Part model, mm, in its own coordinate system. Face numbers are marked on the shaded views. Give positions to 0.01 mm unless a question says otherwise; leave off trailing zeros. Order: outer loops, then holes, each group sorted by start corner. A loop starts at its lowest first (then second) coordinate and runs counter-clockwise, first axis right, second up. Notation, with made-up numbers: M -4.5,-12.5 L 17.5,-12.5 A22 cw 17.5,12.5 Z; hole C -12.75,-33.5 d10. An arc over 180 degrees is marked long. One line per question, with ' | ' between items.
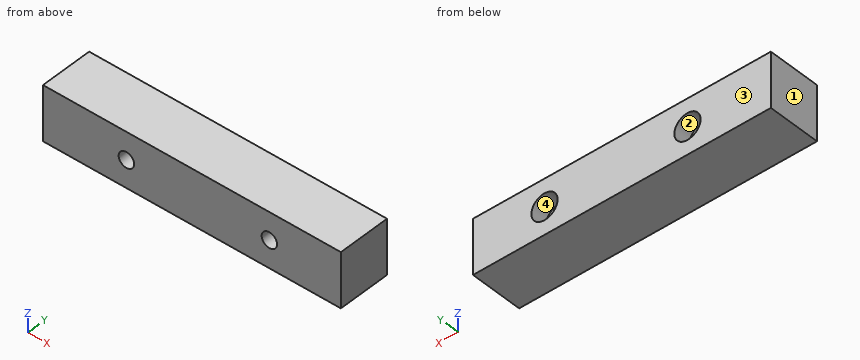
```python
from build123d import *

# Parameters (mm, degrees)
SKETCH_1_W                = 23
SKETCH_1_H                = 22
EXTRUDE_1_DEPTH           = 125
HOLE_WIZARD_1_D           = 6.5
HOLE_WIZARD_1_CBORE_D     = 11
HOLE_WIZARD_1_CBORE_DEPTH = 7
PATTERN_LINEAR_2_COUNT    = 2
PATTERN_LINEAR_2_PITCH    = 60


with BuildPart() as part:
    # 草图1 → 凸台-拉伸1 (new body)
    with BuildSketch(Plane(origin=(0, 0, 0), x_dir=(0, 0, -1), z_dir=(1, 0, 0))):
        Rectangle(SKETCH_1_W, SKETCH_1_H)
    extrude(amount=EXTRUDE_1_DEPTH)

    # 打孔尺寸(%根据)内六角圆柱头螺钉的类型1 (through all)
    with Locations(Plane(origin=(0, 11, 0), x_dir=(1, 0, 0), z_dir=(0, 1, 0))):
        with Locations((35, 0)):
            hole_wizard_1 = CounterBoreHole(HOLE_WIZARD_1_D / 2, HOLE_WIZARD_1_CBORE_D / 2, HOLE_WIZARD_1_CBORE_DEPTH)

    # 阵列(线性)2: 打孔尺寸(%根据)内六角圆柱头螺钉的类型1 ×2
    with Locations(*[(i * PATTERN_LINEAR_2_PITCH, 0, 0) for i in range(1, PATTERN_LINEAR_2_COUNT)]):
        add(hole_wizard_1, mode=Mode.SUBTRACT)


solid = part.part
```
1. Slice it at B-B on y = -5.5. Give the cut face in (x, z), then the cut area to 3 significant figures.
Worked out:
outline: M 0,-11.5 L 125,-11.5 L 125,11.5 L 0,11.5 Z; hole C 35,0 d6.5; hole C 95,0 d6.5 | area: 2,810 mm2
2. Probe L1, parallel to Z at x = 95, y = 9; L2, parallel to X at y = 5.25, z = -4.75; L3, parallel to X at y = -1, z = 0.75. List the from-to ranges inside material, lowest first. Write a range as from..to.
Worked out:
L1: z = -11.5..-5.5, 5.5..11.5 | L2: x = 0..32.23, 37.77..92.23, 97.77..125 | L3: x = 0..31.84, 38.16..91.84, 98.16..125
3. Drop a flat-ended pin along its axis: pin 1 (9 mm diameter, centred on x = 95, z = 0, fed in from +Y). Give the stop position or say it passes through.
Worked out:
pin 1: stops at y = 4
4. Slice it at A-A on z = 0. Give the cut face in (x, y).
Worked out:
outline: M 0,-11 L 31.75,-11 L 31.75,4 L 29.5,4 L 29.5,11 L 0,11 Z; M 38.25,-11 L 91.75,-11 L 91.75,4 L 89.5,4 L 89.5,11 L 40.5,11 L 40.5,4 L 38.25,4 Z; M 98.25,-11 L 125,-11 L 125,11 L 100.5,11 L 100.5,4 L 98.25,4 Z
5. Mould opens along X. For the marked faces 1, 2, 3 and 4 say: released by +X, released by -X, zero draft, split by the parting line, or undercut.
Worked out:
face 1: released by -X | face 2: undercut | face 3: zero draft | face 4: undercut
6. Slice it at C-C on x = 95. Give the cut face in (y, z), then the cut area to 4 significant figures.
Worked out:
outline: M -11,-11.5 L 11,-11.5 L 11,-5.5 L 4,-5.5 L 4,-3.25 L -11,-3.25 Z; M -11,3.25 L 4,3.25 L 4,5.5 L 11,5.5 L 11,11.5 L -11,11.5 Z | area: 331.5 mm2
